The model under review builds one solid part; all positions refer to its coordinate system, in mm. Face numbers are marked on the shaded views. A direction names the side the tool comes from. Coordinates: 2 decimals unless noted, no trailing zeros. Write each loop counter-clockwise with the first axis right and the second up, starting at its lowest first coordinate (ties: lowest second). Pieces come first, ordered by that corner, then holes. Notation, with made-up numbers: (-14.5, 25.5) - (-10.5, 25.5) arc R9 ccw to (-10.5, 42.5) - close; hole circle Ø11 at (87.25, 16.25). An arc over 180 degrees is marked (long way). Put each result on its own line as item: value.
from build123d import *

# Parameters (mm, degrees)
SKETCH1_R           = 75
BOSS_EXTRUDE1_DEPTH = 10
CHAMFER1_SIZE       = 9
SHELL1_T            = -2
SKETCH2_R           = 1.8
CUT_EXTRUDE1_DEPTH  = 107.367288205


with BuildPart() as part:
    # Sketch1 → Boss-Extrude1 (new body)
    with BuildSketch(Plane.XY):
        Circle(SKETCH1_R)
    extrude(amount=BOSS_EXTRUDE1_DEPTH)

    # Chamfer1
    chamfer1_edges = [part.edges().sort_by_distance(p)[0] for p in [
        (-75, 0, 0),
    ]]
    chamfer(chamfer1_edges, length=CHAMFER1_SIZE)

    # Shell1
    shell1_openings = [part.faces().sort_by_distance(p)[0] for p in [
        (0, 0, 10),
    ]]
    offset(amount=SHELL1_T, openings=shell1_openings, kind=Kind.INTERSECTION)

    # Sketch2 → Cut-Extrude1 (cut, through all)
    with BuildSketch(Plane.XY.offset(2)):
        with Locations((2.015078633, 38.755426444)):
            Circle(SKETCH2_R)
        with Locations((-13.325453752, 35.900076006)):
            Circle(SKETCH2_R)
        with Locations((0.548769327, -39.031280101)):
            Circle(SKETCH2_R)
        with Locations((38.672351506, -10.909043386)):
            Circle(SKETCH2_R)
        with Locations((32.346402761, 23.31116451)):
            Circle(SKETCH2_R)
    extrude(amount=-CUT_EXTRUDE1_DEPTH, mode=Mode.SUBTRACT)


solid = part.part
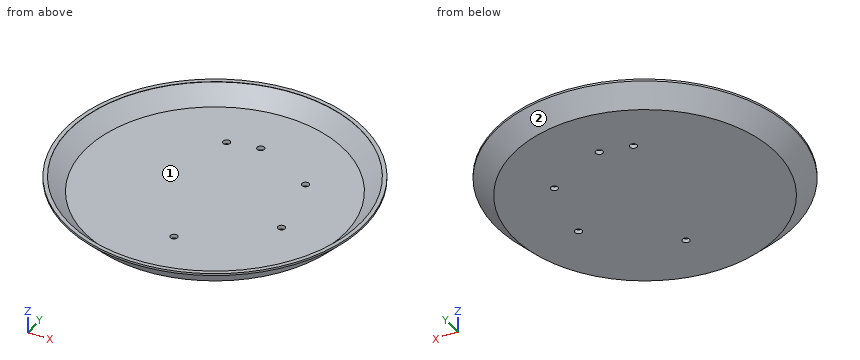
1. Consider section B-B on z = 6.25. State the section outline as (x, y) points, plus the area to 3 significant figures.
Determined:
outline: circle Ø144.5 at (0, 0); hole circle Ø138.84 at (0, 0)
area: 1,260 mm^2
2. Consider section A-A on y = 0. State the section outline as (x, z) points.
Determined:
outline: (-75, 9) - (-66, 0) - (66, 0) - (75, 9) - (75, 10) - (73, 10) - (73, 9.83) - (65.17, 2) - (-65.17, 2) - (-73, 9.83) - (-73, 10) - (-75, 10) - close
3. For pin 1 Ø6 at (x, y) = (0.55, -39.03) entering from +Z; pin 2 Ø2 at (x, y) = (-13.33, 35.9) entering from -Z; pin 3 Ø5 at (y, z) = (11.5, 4.5) entering from +X; pin 4 Ø1.5 at (y, z) = (57.5, 8.5) entering from +X, all flat-tipped, find the tip position at first contact; note any pin that passes through.
Determined:
pin 1: stops at z = 2
pin 2: passes through
pin 3: stops at x = 72.12
pin 4: stops at x = 48.81
4. To check wall thickness, follow probe 1 along Y at (x, z) = (0, 9.9); probe 2 along Z at (x, y) = (-34, -41.5); probe 3 along Y at (x, z) = (-36, 5.25). State the ranges of each line that lie inside material, in increasing order.
Determined:
probe 1: y = -75 to -73, 73 to 75
probe 2: z = 0 to 2
probe 3: y = -61.49 to -58.19, 58.19 to 61.49
5. Machinability: for the marked faces 1 and 2, which of the approach directions +Z, -Z, +X, -X, +Y, -Y give a long, thin tool a straight path to every point of the face, cutting with its end or side? Answer none if there is none.
Determined:
face 1: +Z
face 2: -Z
